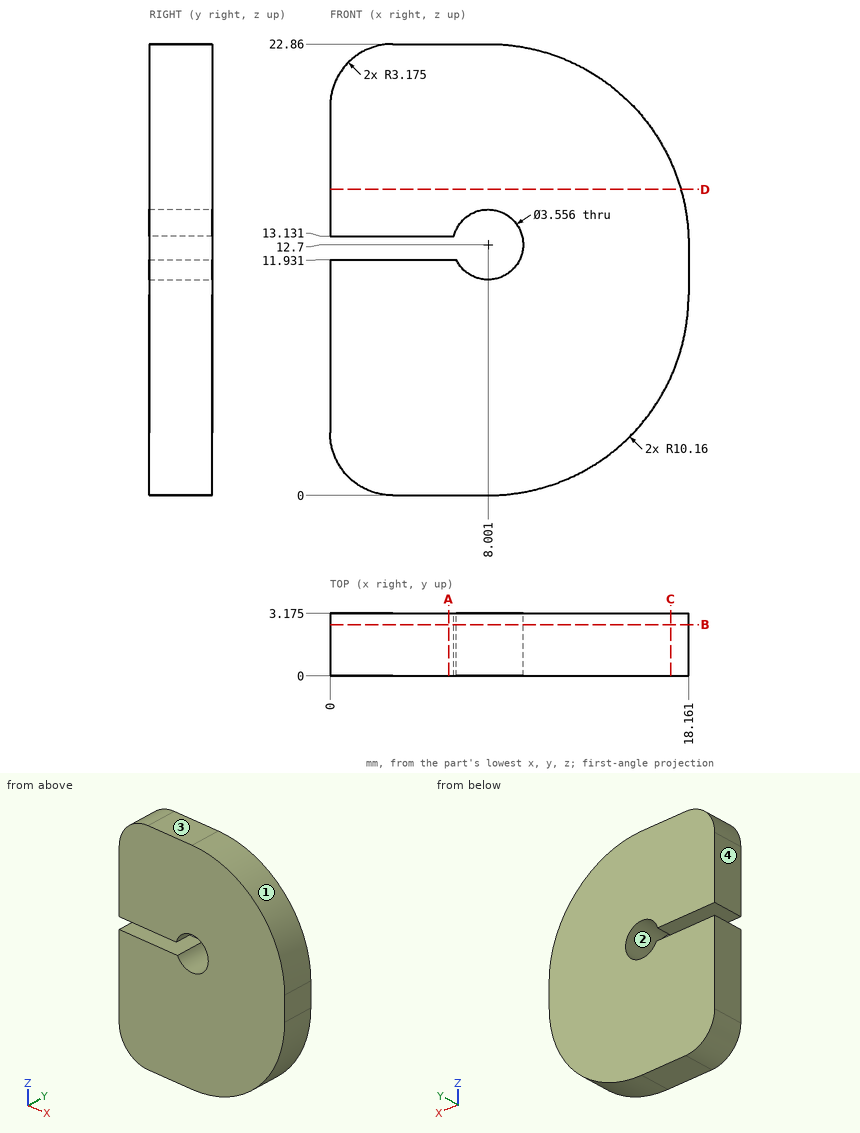
Study the drawing (mm; zero at the part's minimum x, y, z) and answer. Give positions to 0.01 mm unless a question says otherwise; leave off trailing zeros. Write each loop counter-clockwise with the first axis right and the second up, starting at its lowest first coordinate (ties: lowest second). Pieces come first, ordered by that corner, then holes.
(1) The part is cut by section C-C on x = 17.25. Write down the section's boundary in (y, z) (3 decimals), plus the area to 3 significant figures.
Final values:
outline: (0, 5.955) - (3.175, 5.955) - (3.175, 16.905) - (0, 16.905) - close
area: 34.8 mm2
(2) Straight lines are drawn through the part: line 1 (Z direction, x = 8.5, y = 0.25); line 2 (Z direction, x = 9, y = 1.5); line 3 (X direction, y = 1.05, z = 12.75). For each, find the intervals that lie inside material, in ascending order.
Final values:
line 1: z = 0.01 to 10.99, 14.41 to 22.85
line 2: z = 0.05 to 11.23, 14.17 to 22.81
line 3: x = 9.78 to 18.16
(3) The part is cut by section B-B on y = 2.6. Write down the section's boundary in (x, z) (3 decimals).
Final values:
outline: (0, 3.175) arc R3.175 ccw to (3.175, 0) - (8.001, 0) arc R10.16 ccw to (18.161, 10.16) - (18.161, 12.7) arc R10.16 ccw to (8.001, 22.86) - (3.175, 22.86) arc R3.175 ccw to (0, 19.685) - (0, 13.131) - (6.276, 13.131) arc R1.778 cw (long way) to (6.398, 11.931) - (0, 11.931) - close
(4) The mould has two halves that part along X. Classify the marked faces 1, 2, 3 and 4: pulls with the +X half, pulls with the -X half, needs draft (parallel to the pull), parting line crosses it, or undercut.
Final values:
face 1: pulls with the +X half
face 2: undercut
face 3: needs draft
face 4: pulls with the -X half
(5) The part is cut by section A-A on x = 6. Write down the section's boundary in (y, z) (3 decimals), plus the area to 3 significant figures.
Final values:
outline: (0, 0) - (3.175, 0) - (3.175, 11.931) - (0, 11.931) - close; (0, 13.131) - (3.175, 13.131) - (3.175, 22.86) - (0, 22.86) - close
area: 68.8 mm2
(6) The part is cut by section D-D on z = 15.5. Write down the section's boundary in (x, y) (1 decimal), plus the area to 3 significant figures.
Final values:
outline: (0, 0) - (17.8, 0) - (17.8, 3.2) - (0, 3.2) - close
area: 56.4 mm2
